Check sheet for the modelled part. Datum: model origin and axes. Units: mm. Give positions to 0.01 mm unless a question says otherwise; leave off trailing zeros. Write each loop counter-clockwise with the first axis right and the second up, starting at its lowest first coordinate (ties: lowest second). Pieces come first, ordered by that corner, then holes. Notation, with made-up numbers: M 39,-13.5 L 62,-13.5 A25 cw 62,7.5 Z; hole C 26,22.5 d6. An arc over 180 degrees is marked long. Write each question's results on one line, items separated by ' | '. Start each with the question number.
from build123d import *

# Parameters (mm, degrees)
SKETCH1_W           = 196
SKETCH1_H           = 77
BOSS_EXTRUDE1_DEPTH = 58
FILLET1_R           = 7.62
SKETCH2_W           = 2.54
SKETCH2_H           = 7.836102323
SKETCH2_W_2         = 10.16
SKETCH2_H_2         = 2.54
SKETCH2_H_3         = 3.81
SKETCH2_W_3         = 3.81
BOSS_EXTRUDE2_DEPTH = 0.001


with BuildPart() as part:
    # Sketch1 → Boss-Extrude1 (new body)
    with BuildSketch(Plane(origin=(0, 0, 0), x_dir=(1, 0, 0), z_dir=(0, 1, 0))):
        with Locations((98, 38.5)):
            Rectangle(SKETCH1_W, SKETCH1_H)
    extrude(amount=BOSS_EXTRUDE1_DEPTH)

    # Fillet1
    fillet1_edges = [part.edges().sort_by_distance(p)[0] for p in [
        (196, 58, -38.5),
        (98, 58, -77),
        (0, 58, -38.5),
        (98, 0, -77),
        (196, 0, -38.5),
        (98, 0, 0),
        (0, 0, -38.5),
        (0, 29, -77),
        (196, 29, -77),
        (196, 29, 0),
        (0, 29, 0),
        (98, 58, 0),
    ]]
    fillet(fillet1_edges, radius=FILLET1_R)

    # Sketch2 → Boss-Extrude2 (add)
    # profile 1 of 9: a face of its own
    with BuildSketch(Plane.XY):
        with BuildLine():
            Line((139.698967869, 22.283465903), (138.706339513, 24.639564891))
            ThreePointArc((138.706339513, 24.639564891), (136.061823348, 34.079856548), (133.559491145, 24.600884776))
            Line((133.559491145, 24.600884776), (132.489888668, 22.289448892))
            ThreePointArc((132.489888668, 22.289448892), (136.10632402, 36.619997376), (139.698967869, 22.283465903))
        make_face()
    # profile 2 of 9: a face of its own
    with BuildSketch(Plane.XY):
        with Locations((136.1, 23.360894571)):
            Rectangle(SKETCH2_W, SKETCH2_H)
    # profile 3 of 9: a face of its own
    with BuildSketch(Plane.XY):
        with Locations((110.7, 29)):
            Rectangle(SKETCH2_W_2, SKETCH2_H_2)
    # profile 4 of 9: a face of its own
    with BuildSketch(Plane.XY):
        Polygon((88.686666667, 23.134121265), (88.686666667, 34.865878735), (78.526666667, 29), align=None)
        Polygon((82.336666667, 29), (86.781666667, 26.433678053), (86.781666667, 31.566321947), align=None, mode=Mode.SUBTRACT)
    # profile 5 of 9: a face of its own
    with BuildSketch(Plane.XY):
        with Locations((59.9, 32.175)):
            Rectangle(SKETCH2_W, SKETCH2_H_3)
    # profile 6 of 9: a face of its own
    with BuildSketch(Plane.XY):
        with Locations((63.075, 29)):
            Rectangle(SKETCH2_W_3, SKETCH2_H_2)
    # profile 7 of 9: a face of its own
    with BuildSketch(Plane.XY):
        with Locations((59.9, 29)):
            Rectangle(SKETCH2_W, SKETCH2_H_2)
    # profile 8 of 9: a face of its own
    with BuildSketch(Plane.XY):
        with Locations((59.9, 25.825)):
            Rectangle(SKETCH2_W, SKETCH2_H_3)
    # profile 9 of 9: a face of its own
    with BuildSketch(Plane.XY):
        with Locations((56.725, 29)):
            Rectangle(SKETCH2_W_3, SKETCH2_H_2)
    extrude(amount=BOSS_EXTRUDE2_DEPTH)


solid = part.part
Q1. Depth check by flat-ended pin: pin 1 Ø2 at (x, y) = (142.5, 51) entering from +Z. Enter the tip coordinate at first touch or a pass-through.
Q2. Section check B-B on y = 5. Record the boundary of the cut face in (x, z), plus the area to 3 significant figures.
Q3. Section check A-A on y = 54.5. Record the boundary of the cut face in (x, z), plus the area to 3 significant figures.
Q4. Scan lines: L1, parallel to Z at x = 20.5, y = 44.5; L2, parallel to Y at x = 103, z = -7.5; L3, parallel to Y at x = 155.5, z = -70.5. Record each from-to range of solid material in increasing order.
Check result:
1) pin 1: z = 0
2) outline: M 0.46,-69.38 A7.16 ccw 7.62,-76.54 L 188.38,-76.54 A7.16 ccw 195.54,-69.38 L 195.54,-7.62 A7.16 ccw 188.38,-0.46 L 7.62,-0.46 A7.16 ccw 0.46,-7.62 Z | area: 14,800 mm^2
3) outline: M 1.21,-69.38 A6.41 ccw 7.62,-75.79 L 188.38,-75.79 A6.41 ccw 194.79,-69.38 L 194.79,-7.62 A6.41 ccw 188.38,-1.21 L 7.62,-1.21 A6.41 ccw 1.21,-7.62 Z | area: 14,400 mm^2
4) L1: -77 to 0 | L2: 0 to 58 | L3: 0.08 to 57.92
